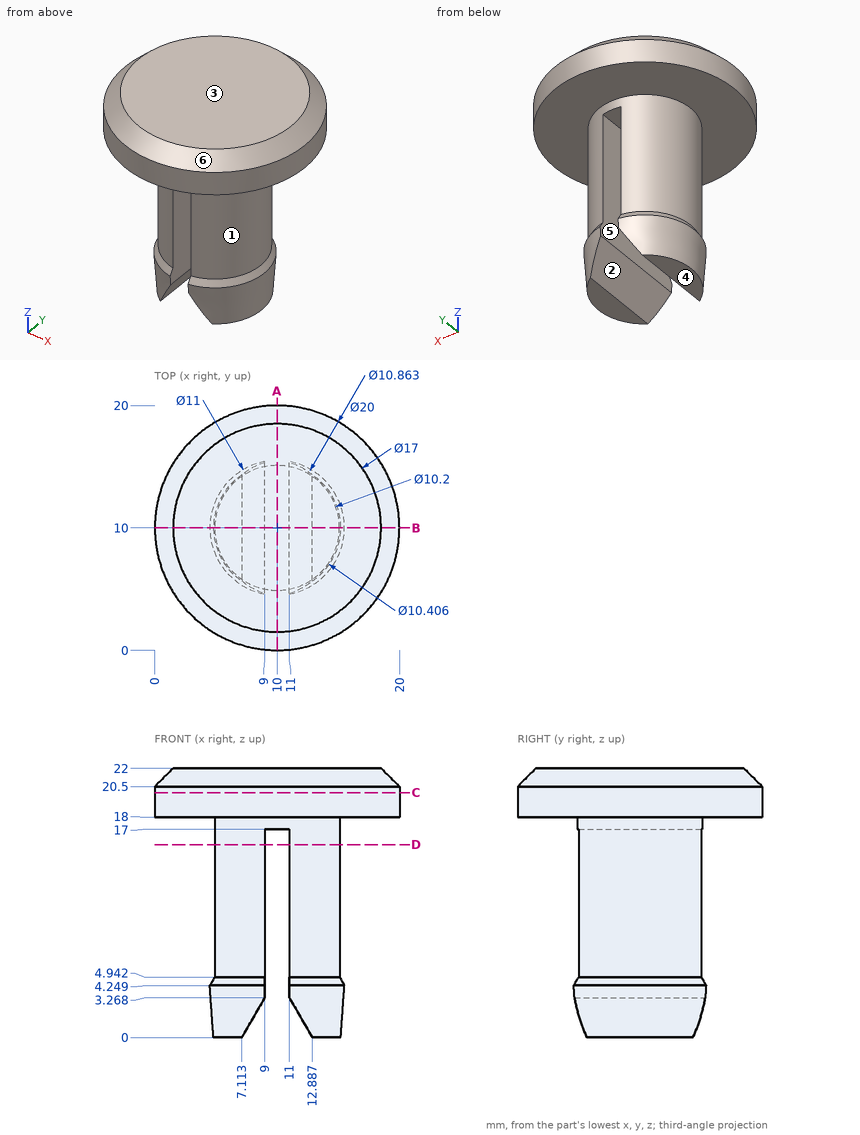
Source: three-view drawing plus pictorial views. Frame: mm from the lowest corner of the part. A direction names the side the tool comes from. Give positions to 0.01 mm unless a question says otherwise; leave off trailing zeros. Loops run counter-clockwise (first coordinate to the right, second up) from the corner with the lowest first, then second, coordinate; pieces in that order, holes last.
1) Section query B-B on y = 10. Return the cut outline in (x, z).
A:
outline: (0, 18) - (4.9, 18) - (4.9, 4.94) - (4.5, 4.25) - (4.8, 0) - (7.11, 0) - (9, 3.27) - (9, 17) - (11, 17) - (11, 3.27) - (12.89, 0) - (15.2, 0) - (15.5, 4.25) - (15.1, 4.94) - (15.1, 18) - (20, 18) - (20, 20.5) - (18.5, 22) - (1.5, 22) - (0, 20.5) - close
2) Section query A-A on x = 10. Return the cut outline in (y, z).
A:
outline: (0, 18) - (4.9, 18) - (4.9, 17) - (15.1, 17) - (15.1, 18) - (20, 18) - (20, 20.5) - (18.5, 22) - (1.5, 22) - (0, 20.5) - close
3) Section query C-C on z = 20. Return the cut outline in (x, y).
A:
outline: circle Ø20 at (10, 10)
4) Section query D-D on z = 15.75. Return the cut outline in (x, y).
A:
outline: (9, 5) - (9, 15) arc R5.1 ccw to start; (11, 5) arc R5.1 ccw to (11, 15) - close
5) Contact query for flat-ended pins moving along their axis: pin 1 (1.5 mm diameter, centred on y = 6.5, z = 5, fed in from +X); pin 2 (2 mm diameter, centred on x = 8.5, y = 11, fed in from -Z); pin 3 (3 mm diameter, centred on y = 12.5, z = 12.5, fed in from -X); pin 4 (10 mm diameter, centred on x = 8.5, y = 12, fed in from -Z). Output: stop coordinate, or through.
A:
pin 1: stops at x = 14.48
pin 2: stops at z = 0.67
pin 3: stops at x = 5
pin 4: stops at z = 0
6) Mould query, pull axis X, two halves, no side actions, for the marked faces 4, 5 and 6. Classes: released by +X, released by -X, zero draft, split by the parting line, or undercut.
A:
face 4: zero draft
face 5: undercut
face 6: split by the parting line
7) Line query: L1, parallel to Z at x = 13.25, y = 5.5; L2, parallel to Z at x = 10.25, y = 8.5; L3, parallel to X at y = 9, z = 11.5. Output: solid intervals per line, ascending.
A:
L1: z = 18 to 22
L2: z = 17 to 22
L3: x = 5 to 9, 11 to 15
8) Reachability of the marked faces 1, 2 and 3 from +Z, -Z, +X, -X, +Y, -Y: full face, straight path, thin tool, end or side. Return the list, or none.
A:
face 1: none
face 2: -Z, +Y, -Y
face 3: +Z, +X, -X, +Y, -Y
